Can you work these out from the model? Positions are in its coordinate system, mm. Face numbers are marked on the shaded views. A direction names the side the tool comes from. Give positions to 0.01 mm unless a question says otherwise; leave off trailing zeros. Loops run counter-clockwise (first coordinate to the right, second up) from the corner with the lowest first, then second, coordinate; pieces in that order, holes last. Notation, with made-up numbers: M 76,28.25 L 125,28.25 A21 cw 125,50.25 Z; hole C 77,-29.5 d5. An arc over 180 degrees is marked long. Answer as a JSON object with one key per item and string values.
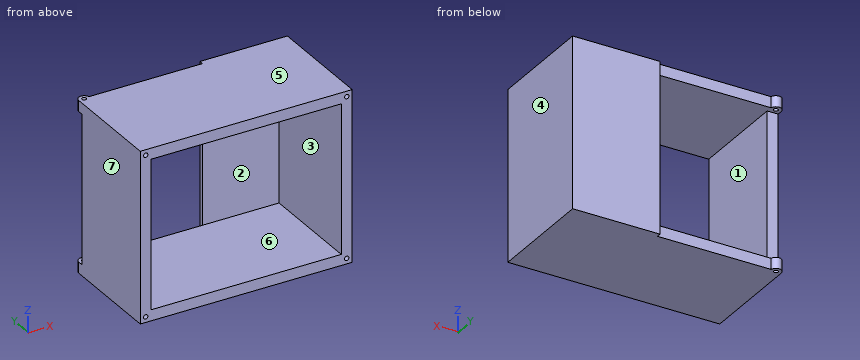
```python
from build123d import *

# Parameters (mm, degrees)
SKETCH1_W               = 80
SKETCH1_H               = 5
BOSS_EXTRUDE1_DEPTH     = 156
SKETCH2_W               = 174
SKETCH2_H               = 136
CUT_EXTRUDE1_DEPTH      = 96
SKETCH3_W               = 94
SKETCH3_H               = 136
CUT_EXTRUDE2_DEPTH      = 96
SKETCH6_W               = 10
SKETCH6_H               = 5
CUT_EXTRUDE3_DEPTH      = 136
CUT_EXTRUDE4_DEPTH      = 183.277261336
CUT_EXTRUDE4_DEPTH_BACK = 183.277261336
SKETCH7_W               = 114
SKETCH7_H               = 4
CUT_EXTRUDE9_REACH      = 192.381
BOSS_EXTRUDE2_DEPTH     = 10
SKETCH10_R              = 2
CUT_EXTRUDE10_DEPTH     = 96
SKETCH12_R              = 2
CUT_EXTRUDE11_DEPTH     = 60


with BuildPart() as part:
    # Sketch1 → Boss-Extrude1 (new body)
    with BuildSketch(Plane.XY):
        Polygon((-97, 50), (-97, -50), (97, -50), (97, 45), (17, 45), (17, 50), align=None)
        with Locations((57, 47.5)):
            Rectangle(SKETCH1_W, SKETCH1_H)
    extrude(amount=BOSS_EXTRUDE1_DEPTH)

    # Sketch2 → Cut-Extrude1 (cut)
    with BuildSketch(Plane(origin=(0, -50, 0), x_dir=(-1, 0, 0), z_dir=(0, -1, 0))):
        with Locations((0, -78)):
            Rectangle(SKETCH2_W, SKETCH2_H)
    extrude(amount=-CUT_EXTRUDE1_DEPTH, mode=Mode.SUBTRACT)

    # Sketch3 → Cut-Extrude2 (cut)
    with BuildSketch(Plane(origin=(0, 50, 0), x_dir=(1, 0, 0), z_dir=(0, 1, 0))):
        with Locations((-40, -78)):
            Rectangle(SKETCH3_W, SKETCH3_H)
    extrude(amount=-CUT_EXTRUDE2_DEPTH, mode=Mode.SUBTRACT)

    # Sketch6 → Cut-Extrude3 (cut)
    with BuildSketch(Plane.XY.offset(10)):
        with Locations((12, 47.5)):
            Rectangle(SKETCH6_W, SKETCH6_H)
    extrude(amount=CUT_EXTRUDE3_DEPTH, mode=Mode.SUBTRACT)

    # Sketch7 → Cut-Extrude4 (cut, two sides: drawn at the far end of the back side and taken through both)
    with BuildSketch(Plane.XY.offset(10).offset(-CUT_EXTRUDE4_DEPTH_BACK)):
        with Locations((-40, 48)):
            Rectangle(SKETCH7_W, SKETCH7_H)
    extrude(amount=CUT_EXTRUDE4_DEPTH + CUT_EXTRUDE4_DEPTH_BACK, mode=Mode.SUBTRACT)

    # Cut-Extrude9: up to this face of the body (flat: up to its plane)
    cut_extrude9_end = Plane(part.part.faces().sort_by_distance((0.962837838, -1.155405405, 156))[0])
    # Sketch8 → Cut-Extrude9 (cut, up to the picked face)
    with BuildSketch(Plane.XY, mode=Mode.PRIVATE) as cut_extrude9_sk1:
        Polygon((-97, 46), (-97, 45), (-97, 40), (-92, 40), (-87, 40), (-87, 46), align=None)
    cut_extrude9_tool1 = split(extrude(cut_extrude9_sk1.sketch, amount=CUT_EXTRUDE9_REACH, mode=Mode.PRIVATE), bisect_by=cut_extrude9_end, keep=Keep.BOTH, mode=Mode.PRIVATE)
    add(cut_extrude9_tool1.solids().sort_by(Axis((-92, 43, 0), (0, 0, 1)))[0], mode=Mode.SUBTRACT)

    # Sketch9 → Boss-Extrude2 (add)
    with BuildSketch(Plane.XY.offset(156)):
        with BuildLine():
            Line((-97, 40), (-97, 45))
            ThreePointArc((-97, 45), (-92.50254481, 49.974680765), (-87.101020514, 46))
            Line((-87.101020514, 46), (-87, 46))
            Line((-87, 46), (-87, 45))
            Line((-87, 45), (-87, 40))
            Line((-87, 40), (-97, 40))
        make_face()
    boss_extrude2 = extrude(amount=-BOSS_EXTRUDE2_DEPTH)

    # Sketch10 → Cut-Extrude10 (cut)
    with BuildSketch(Plane(origin=(0, 0, 146), x_dir=(-1, 0, 0), z_dir=(0, 0, -1))):
        with Locations((92, 45)):
            Circle(SKETCH10_R)
    cut_extrude10 = extrude(amount=-CUT_EXTRUDE10_DEPTH, mode=Mode.SUBTRACT)

    # Mirror1: Boss-Extrude2, Cut-Extrude10 across plane
    add(boss_extrude2.mirror(Plane.XY.offset(78)))
    add(cut_extrude10.mirror(Plane.XY.offset(78)), mode=Mode.SUBTRACT)

    # Sketch12 → Cut-Extrude11 (cut)
    with BuildSketch(Plane(origin=(0, -50, 0), x_dir=(-1, 0, 0), z_dir=(0, -1, 0))):
        with Locations(Location((92, -151, 0), (0, 0, 90))):
            Circle(SKETCH12_R)
        with Locations(Location((-92, -151, 0), (0, 0, 90))):
            Circle(SKETCH12_R)
        with Locations(Location((-92, -5, 0), (0, 0, 90))):
            Circle(SKETCH12_R)
        with Locations(Location((92, -5, 0), (0, 0, 90))):
            Circle(SKETCH12_R)
    extrude(amount=-CUT_EXTRUDE11_DEPTH, mode=Mode.SUBTRACT)


solid = part.part
```
1) For the marked faces 1, 2, 3 and 4, which set-ups out of +Z, -Z, +X, -X, +Y, -Y let a thin tool reach every point of the face, with its end or its side?
Answer list:
{"face 1": "+Y, -Y", "face 2": "-X, -Y", "face 3": "-Y", "face 4": "+Z, -Z, +X, +Y, -Y"}
2) Suppose I cut it at D-D, the plane x = 22. Write out the boundary of the cut face in (y, z).
Answer list:
{"outline": "M -50,0 L 50,0 L 50,156 L -50,156 L -50,146 L 46,146 L 46,10 L -50,10 Z"}
3) Will these pins go through, and if not, where does the flat tip stop? pin 1 Ø4 at (x, y) = (30.5, 29.5) entering from -Z; pin 2 Ø1.2 at (x, z) = (91, 151) entering from -Y; pin 3 Ø8 at (x, z) = (24.5, 17) entering from -Y; pin 4 Ø4.5 at (y, z) = (48.5, 94) entering from -X.
Answer list:
{"pin 1": "z = 0", "pin 2": "y = 10", "pin 3": "y = 46", "pin 4": "x = 17"}
4) Please list where these lines run through material, in increasing order: line 1 along X through (y, z) = (-26, 151); line 2 along Z through (x, y) = (-45.5, 19.5); line 3 along X through (y, z) = (2, 33). Write a range as from..to.
Answer list:
{"line 1": "-97..-94, -90..90, 94..97", "line 2": "0..10, 146..156", "line 3": "-97..-87, 87..97"}
5) Suppose I cut it at B-B, the plane z = 86.5. Write out the boundary of the cut face in (x, y).
Answer list:
{"outline": "M -97,-50 L -87,-50 L -87,40 L -97,40 Z; M 17,46 L 87,46 L 87,-50 L 97,-50 L 97,50 L 17,50 Z"}
6) Suppose I cut it at A-A, the plane x = -51. Write out the boundary of the cut face in (y, z).
Answer list:
{"outline": "M -50,0 L 46,0 L 46,10 L -50,10 Z; M -50,146 L 46,146 L 46,156 L -50,156 Z"}
7) If we mould it in two halves opening along X, with no side actions, what happens to the marked faces 5, 6 and 7? For each: +X half, -X half, draft (parallel to the pull), parting line (faces both ways), or undercut.
Answer list:
{"face 5": "draft", "face 6": "undercut", "face 7": "-X half"}
8) Suppose I cut it at C-C, the plane y = 19.5. Write out the boundary of the cut face in (x, z).
Answer list:
{"outline": "M -97,0 L 97,0 L 97,156 L -97,156 Z; hole M -87,10 L 87,10 L 87,146 L -87,146 Z"}
